Verification items for this drawing (mm, ordinates from the low corner). Coordinates: 2 decimals unless noted, no trailing zeros. Order: outer loops, then holes, each group sorted by start corner. A loop starts at its lowest first (then second) coordinate and runs counter-clockwise, first axis right, second up. Notation, with made-up numbers: M 85,83 L 127,83 A22 ccw 127,101 Z; hole C 35,41.5 d2. An arc over 180 degrees is marked long. Answer as a JSON object with one key per item and string values. Group by question number.
(1) Cross-section at B-B (x = 71). Enter the section's corners in (y, z), plus the area to 3 significant figures.
(2) Material ranges on line 1 (Z direction, x = 35.5, y = 1.35); line 2 (X direction, y = 1.1, z = 6.75); line 3 (X direction, y = 1.45, z = 9), recorded low to high.
(3) Cross-section at A-A (y = 0.65). Enter the section's corners in (x, z).
(4) Cross-section at C-C (z = 2.25). Enter the section's corners in (x, y), plus the area to 3 significant figures.
(5) Gauge pin test, flat ends, axial feed: pin 1 Ø1.3 at (x, y) = (26, 1.5) entering from -Z; pin 2 Ø1.3 at (y, z) = (1, 10.5) entering from -X; pin 3 Ø1.5 at (x, y) = (83, 1.5) entering from -Z; pin 4 Ø0.8 at (y, z) = (1, 10) entering from +X. Record the tip position at first contact, or that the pin passes through.
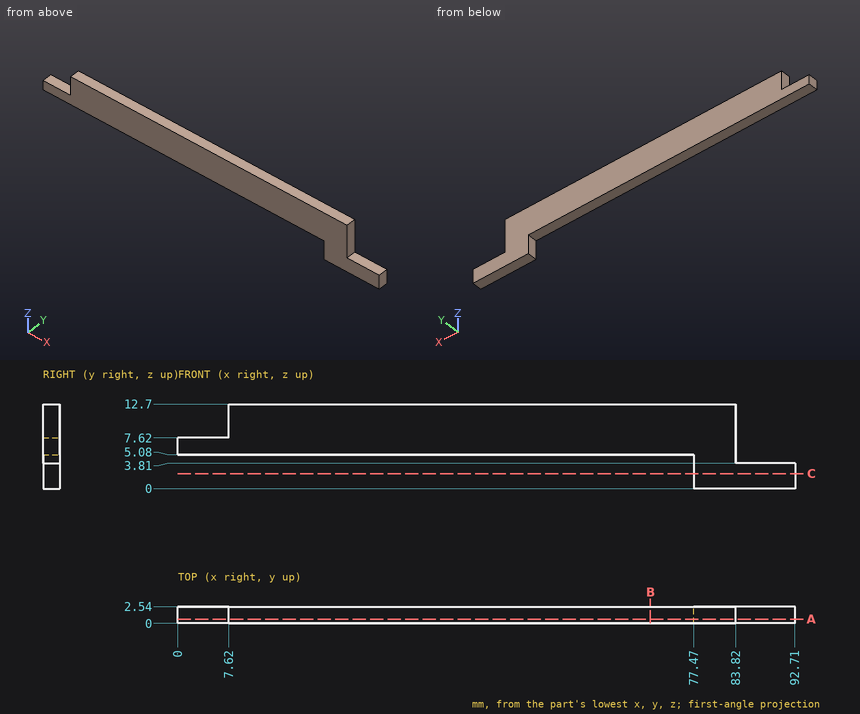
Taken from the geometry:
{
 "1": {"outline": "M 0,5.08 L 2.54,5.08 L 2.54,12.7 L 0,12.7 Z", "area": "19.4 mm²"},
 "2": {"line 1": "z = 5.08 to 12.7", "line 2": "x = 0 to 83.82", "line 3": "x = 7.62 to 83.82"},
 "3": {"outline": "M 0,5.08 L 77.47,5.08 L 77.47,0 L 92.71,0 L 92.71,3.81 L 83.82,3.81 L 83.82,12.7 L 7.62,12.7 L 7.62,7.62 L 0,7.62 Z"},
 "4": {"outline": "M 77.47,0 L 92.71,0 L 92.71,2.54 L 77.47,2.54 Z", "area": "38.7 mm²"},
 "5": {"pin 1": "stops at z = 5.08", "pin 2": "stops at x = 7.62", "pin 3": "stops at z = 0", "pin 4": "stops at x = 83.82"}
}
